from build123d import *

# Parameters (mm, degrees)
DODANIE_WYCI_GNI_CIE1_DEPTH = 70
SKORUPA1_T                  = -1.5
SZKIC2_W                    = 2
SZKIC2_H                    = 6
DODANIE_WYCI_GNI_CIE2_DEPTH = 50
ZAOKR_GLENIE2_R             = 1


with BuildPart() as part:
    # Szkic1 → Dodanie-wyciągnięcie1 (new body)
    with BuildSketch(Plane(origin=(0, 0, 0), x_dir=(1, 0, 0), z_dir=(0, 1, 0))):
        with BuildLine():
            Line((-5.5, 4.5), (5.5, 4.5))
            ThreePointArc((5.5, 4.5), (10, 0), (5.5, -4.5))
            Line((5.5, -4.5), (-5.5, -4.5))
            ThreePointArc((-5.5, -4.5), (-10, 0), (-5.5, 4.5))
        make_face()
    extrude(amount=DODANIE_WYCI_GNI_CIE1_DEPTH)

    # Skorupa1
    skorupa1_openings = [part.faces().sort_by_distance(p)[0] for p in [
        (0, 70, 0),
    ]]
    offset(amount=SKORUPA1_T, openings=skorupa1_openings, kind=Kind.INTERSECTION)

    # Szkic2 → Dodanie-wyciągnięcie2 (add)
    with BuildSketch(Plane(origin=(0, 1.5, 0), x_dir=(1, 0, 0), z_dir=(0, 1, 0))):
        Rectangle(SZKIC2_W, SZKIC2_H)
    extrude(amount=DODANIE_WYCI_GNI_CIE2_DEPTH)

    # Zaokrąglenie2
    zaokr_glenie2_edges = [part.edges().sort_by_distance(p)[0] for p in [
        (0, 0, -4.5),
        (10, 0, 0),
        (0, 0, 4.5),
        (-10, 0, 0),
        (-1, 51.5, 0),
        (1, 51.5, 0),
    ]]
    fillet(zaokr_glenie2_edges, radius=ZAOKR_GLENIE2_R - 0.0001)  # a hair under: the kernel refuses the full size


solid = part.part
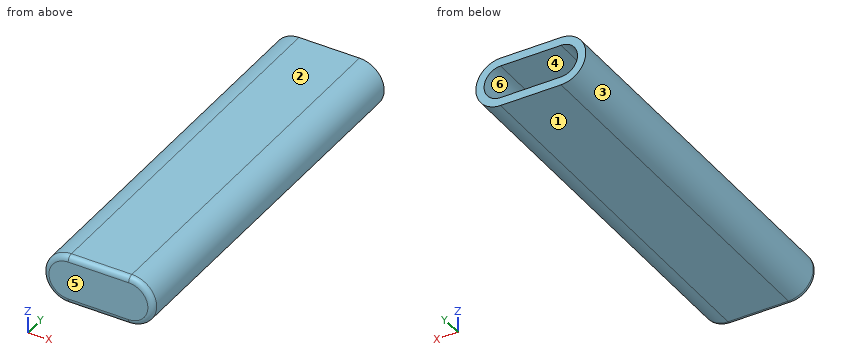
Verification items for the finished model (mm, model axes). Face numbers are marked on the shaded views. A direction names the side the tool comes from. Give positions to 0.01 mm unless a question says otherwise; leave off trailing zeros. Loops run counter-clockwise (first coordinate to the right, second up) from the corner with the lowest first, then second, coordinate; pieces in that order, holes last.
1) Set-up check for the marked faces 5 and 6: record each of +Z, -Z, +X, -X, +Y, -Y from which the full face is reachable in a straight line by a thin tool's end or side.
2) Depth check by flat-ended pin: pin 1 Ø2 at (y, z) = (15.5, 2) entering from +X; pin 2 Ø3 at (x, z) = (4, 0) entering from +Y. Enter the tip coordinate at first touch or a pass-through.
3) Draft check along Z on the marked faces 1, 2, 3 and 4. Enter one of: pulls with the +Z half, pulls with the -Z half, needs draft (parallel to the pull), parting line crosses it, or undercut.
4) Sectioned sample at A-A, the plane y = 17.5. Enter the section's corners in (x, z), then the cut area to 3 significant figures.
5) Sectioned sample at B-B, the plane x = -2.75. Enter the section's corners in (y, z).
6) Thickness scan on line 1 along X through (y, z) = (37.5, 0); line 2 along Z through (x, y) = (1, 57); line 3 along X through (y, z) = (27, -1.75). Record the ranges inside material, lowest first.
Answers:
1. face 5: +Z, -Z, +X, -X, -Y
1. face 6: +Y
2. pin 1: stops at x = 9.89
2. pin 2: stops at y = 1.5
3. face 1: pulls with the -Z half
3. face 2: pulls with the +Z half
3. face 3: parting line crosses it
3. face 4: undercut
4. outline: (-5.5, -4.5) - (5.5, -4.5) arc R4.5 ccw to (5.5, 4.5) - (-5.5, 4.5) arc R4.5 ccw to start; hole (-5.5, -3) - (-1, -3) - (-1, 3) - (-5.5, 3) arc R3 ccw to start; hole (1, -3) - (5.5, -3) arc R3 ccw to (5.5, 3) - (1, 3) - close
4. area: 80.3 mm2
5. outline: (0, -3.5) arc R1 ccw to (1, -4.5) - (70, -4.5) - (70, -3) - (1.5, -3) - (1.5, 3) - (70, 3) - (70, 4.5) - (1, 4.5) arc R1 ccw to (0, 3.5) - close
6. line 1: x = -10 to -8.5, -1 to 1, 8.5 to 10
6. line 2: z = -4.5 to -3, 3 to 4.5
6. line 3: x = -9.65 to -7.94, -1 to 1, 7.94 to 9.65
